Verification items for the finished model (mm, model axes). Face numbers are marked on the shaded views. A direction names the side the tool comes from. Give positions to 0.01 mm unless a question says otherwise; leave off trailing zeros. Order: outer loops, then holes, each group sorted by start corner. A loop starts at its lowest first (then second) coordinate and runs counter-clockwise, first axis right, second up. Notation, with made-up numbers: (-32, 39.25) -> (12, 39.25) arc R18 ccw to (12, 61.25) -> close; hole circle Ø6 at (-3.5, -29). An arc over 180 degrees is marked (long way). Return JSON: item names as keys, results as strings. Group by question number.
(1) Cross-section at B-B on y = 4.5. Enter the section's corners in (x, z).
(2) Cross-section at D-D on z = 7.5. Enter the section's corners in (x, y).
(3) Thickness scan on line 1 along Y through (x, z) = (-39.5, 2.5); line 2 along X through (y, z) = (0, 25); line 3 along Z through (x, y) = (30, 11). Record the ranges inside material, lowest first.
(4) Tool access check on the marked faces 1 and 2. Record the directions out of +Z, -Z, +X, -X, +Y, -Y that give a thin tool (end or side, any length) a straight path to the whole face; none if there is none.
(5) Depth check by flat-ended pin: pin 1 Ø3 at (x, y) = (0.5, -1.5) entering from +Z; pin 2 Ø5.5 at (x, z) = (0, 29.25) entering from -Y; pin 3 Ø10 at (y, z) = (8.5, 7) entering from -X; pin 4 Ø4 at (x, y) = (34.5, 3) entering from -Z. Enter the tip coordinate at first touch or a pass-through.
(6) Cross-section at C-C on x = -4.5. Enter the section's corners in (y, z), then the cut area to 3 significant figures.
(7) Cross-section at A-A on y = 0. Enter the section's corners in (x, z), then the cut area to 3 significant figures.
from build123d import *

# Parameters (mm, degrees)
CROQUIS1_R                 = 5.85
SALIENTE_EXTRUIR1_DEPTH    = 38
CROQUIS2_R                 = 1.75
CORTAR_EXTRUIR1_DEPTH      = 7.5
CROQUIS3_R                 = 45
SALIENTE_EXTRUIR2_DEPTH    = 3.2
CORTAR_EXTRUIR2_DEPTH      = 75.121521892
CORTAR_EXTRUIR2_DEPTH_BACK = 5
CROQUIS5_R                 = 3.65


with BuildPart() as part:
    # Croquis1 → Saliente-Extruir1 (new body)
    with BuildSketch(Plane.XY):
        Circle(CROQUIS1_R)
        with BuildLine():
            Line((-1.8, 2.585053191), (1.8, 2.585053191))
            ThreePointArc((1.8, 2.585053191), (0, -3.15), (-1.8, 2.585053191))
        make_face(mode=Mode.SUBTRACT)
    extrude(amount=SALIENTE_EXTRUIR1_DEPTH)

    # Croquis2 → Cortar-Extruir1 (cut)
    with BuildSketch(Plane(origin=(0, 2.585053191, 0), x_dir=(1, 0, 0), z_dir=(0, 1, 0))):
        with Locations((0, -34.75)):
            Circle(CROQUIS2_R)
        with Locations((0, -29.25)):
            Circle(CROQUIS2_R)
    extrude(amount=CORTAR_EXTRUIR1_DEPTH, mode=Mode.SUBTRACT)

    # Croquis3 → Saliente-Extruir2 (add)
    with BuildSketch(Plane(origin=(0, 0, 0), x_dir=(-1, 0, 0), z_dir=(0, 0, -1))):
        Circle(CROQUIS3_R)
    extrude(amount=-SALIENTE_EXTRUIR2_DEPTH)

    # Croquis5 → Cortar-Extruir2 (cut, two sides: drawn at the far end of the back side and taken through both)
    with BuildSketch(Plane(origin=(0, 0, 0), x_dir=(-1, 0, 0), z_dir=(0, 0, -1)).offset(-CORTAR_EXTRUIR2_DEPTH_BACK)):
        with Locations(Location((-39.5, 0, 0), (0, 0, 180))):
            Circle(CROQUIS5_R)
        with Locations(Location((39.5, 0, 0), (0, 0, 180))):
            Circle(CROQUIS5_R)
        Polygon((0, 20), (-75, 20), (-75, 50), (75, 50), (75, 20), align=None)
        Polygon((75, -50), (75, -20), (0, -20), (-75, -20), (-75, -50), align=None)
    extrude(amount=CORTAR_EXTRUIR2_DEPTH + CORTAR_EXTRUIR2_DEPTH_BACK, mode=Mode.SUBTRACT)


solid = part.part
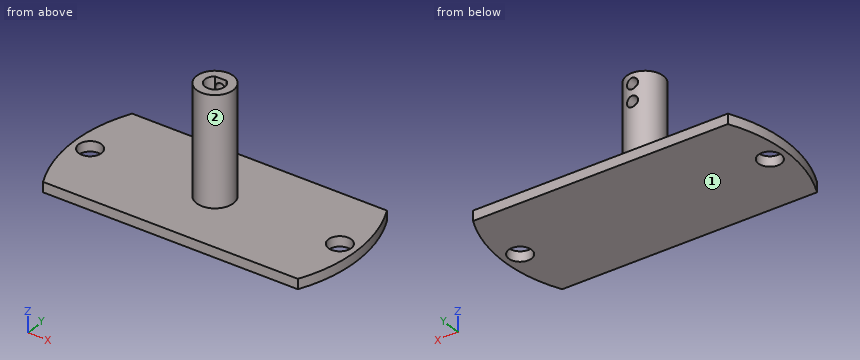
Verdict:
{
 "1": {"outline": "(-44.77, 0) -> (44.77, 0) -> (44.77, 3.2) -> (3.74, 3.2) -> (3.74, 38) -> (-3.74, 38) -> (-3.74, 3.2) -> (-44.77, 3.2) -> close; hole circle Ø3.5 at (0, 29.25); hole circle Ø3.5 at (0, 34.75)"},
 "2": {"outline": "circle Ø11.7 at (0, 0); hole (-1.8, 2.59) arc R3.15 ccw (long way) to (1.8, 2.59) -> close"},
 "3": {"line 1": "-20 to -3.65, 3.65 to 20", "line 2": "-5.85 to -3.15, 3.15 to 5.85", "line 3": "0 to 3.2"},
 "4": {"face 1": "-Z, +X, -X, +Y, -Y", "face 2": "+Z"},
 "5": {"pin 1": "z = 3.2", "pin 2": "y = -5.85", "pin 3": "x = -44.69", "pin 4": "z = 0"},
 "6": {"outline": "(-20, 0) -> (20, 0) -> (20, 3.2) -> (3.74, 3.2) -> (3.74, 38) -> (-3.74, 38) -> (-3.74, 3.2) -> (-20, 3.2) -> close", "area": "388 mm²"},
 "7": {"outline": "(-45, 0) -> (-43.15, 0) -> (-43.15, 3.2) -> (-45, 3.2) -> close; (-35.85, 0) -> (35.85, 0) -> (35.85, 3.2) -> (5.85, 3.2) -> (5.85, 38) -> (3.15, 38) -> (3.15, 3.2) -> (-3.15, 3.2) -> (-3.15, 38) -> (-5.85, 38) -> (-5.85, 3.2) -> (-35.85, 3.2) -> close; (43.15, 0) -> (45, 0) -> (45, 3.2) -> (43.15, 3.2) -> close", "area": "429 mm²"}
}
